from build123d import *

# Parameters (mm, degrees)
BOSS_EXTRUDE1_DEPTH = 17.5
SKETCH2_R           = 1.175
CUT_EXTRUDE1_DEPTH  = 4.41
SKETCH3_R           = 2.75
CUT_EXTRUDE2_DEPTH  = 1


with BuildPart() as part:
    # Sketch1 → Boss-Extrude1 (new body, symmetric)
    with BuildSketch(Plane.XY):
        with BuildLine():
            Line((-3.14, 0.055), (-3.14, -0.055))
            ThreePointArc((-3.14, -0.055), (-3.476827202, -0.868172798), (-4.29, -1.205))
            Line((-4.29, -1.205), (-4.29, -1.705))
            Line((-4.29, -1.705), (4.29, -1.705))
            Line((4.29, -1.705), (4.29, -1.205))
            ThreePointArc((4.29, -1.205), (3.476827202, -0.868172798), (3.14, -0.055))
            Line((3.14, -0.055), (3.14, 0.055))
            ThreePointArc((3.14, 0.055), (3.476827202, 0.868172798), (4.29, 1.205))
            Line((4.29, 1.205), (4.29, 1.705))
            Line((4.29, 1.705), (-4.29, 1.705))
            Line((-4.29, 1.705), (-4.29, 1.205))
            ThreePointArc((-4.29, 1.205), (-3.476827202, 0.868172798), (-3.14, 0.055))
        make_face()
    extrude(amount=BOSS_EXTRUDE1_DEPTH, both=True)

    # Sketch2 → Cut-Extrude1 (cut, through all)
    with BuildSketch(Plane(origin=(0, 1.705, 0), x_dir=(1, 0, 0), z_dir=(0, 1, 0))):
        with Locations((0, 12.5)):
            Circle(SKETCH2_R)
    cut_extrude1 = extrude(amount=-CUT_EXTRUDE1_DEPTH, mode=Mode.SUBTRACT)

    # Sketch3 → Cut-Extrude2 (cut)
    with BuildSketch(Plane(origin=(0, 1.705, 0), x_dir=(1, 0, 0), z_dir=(0, 1, 0))):
        with Locations((0, 12.5)):
            Circle(SKETCH3_R)
    cut_extrude2 = extrude(amount=-CUT_EXTRUDE2_DEPTH, mode=Mode.SUBTRACT)

    # Mirror1: Cut-Extrude1, Cut-Extrude2 across plane
    add(cut_extrude1.mirror(Plane.XY), mode=Mode.SUBTRACT)
    add(cut_extrude2.mirror(Plane.XY), mode=Mode.SUBTRACT)


solid = part.part
Verification items for the finished model (mm, model axes). A direction names the side the tool comes from. Round coordinates to 2 decimals unless told otherwise and drop trailing zeros. Loops run counter-clockwise (first coordinate to the right, second up) from the corner with the lowest first, then second, coordinate; pieces in that order, holes last. Notation, with made-up numbers: (64.5, 28) - (74.5, 28) arc R24 ccw to (74.5, 47) - close; hole circle Ø10 at (49.5, 79). An arc over 180 degrees is marked (long way). Use a Markdown table: item, result. Add a question column.
1. Release check for a two-part mould opening along X. For faces 6 (the face through (0, -1.705, 0)), 7 (the face through (-0.25, -0.48, 11.35)), 8 (the face through (-3.47, -0.86, 0.25)) record: released by +X, released by -X, zero draft, split by the parting line, or undercut.
2. Section check A-A, the plane x = 0. Record the boundary of the cut face in (y, z) (3 decimals).
3. Thickness scan on probe 1 along Z at (x, y) = (0, -0.45) (3 decimals); probe 2 along Z at (x, y) = (0, 1.15); probe 3 along X at (y, z) = (-0.15, 2). Record the ranges inside material, lowest first. Write a range as [from, to].
4. Section check B-B, the plane z = 12.5. Record the boundary of the cut face in (x, y) (3 decimals).
5. Section check D-D, the plane z = 7.5. Record the boundary of the cut face in (x, y) (3 decimals).
6. Section check C-C, the plane y = -0.5. Record the boundary of the cut face in (x, z) (3 decimals).
7. Access from +Z, -Z, +X, -X, +Y, -Y to the whole of each face (thin tool, end or side, straight path). Record for faces 1 (the face through (0, 0.705, -11)), 2 (the face through (0, 1.705, 0)), 3 (the face through (-3.49, 0.88, 0.25)), 4 (the face through (3.47, 0.86, 0.25)), 5 (the face through (-0.25, -0.48, -11.35)).
8. Gauge pin test, flat ends, axial feed: pin 1 (5 mm diameter, centred on x = 0, z = -12.5, fed in from +Y) (3 decimals); pin 2 (1 mm diameter, centred on y = 0, z = 12.5, fed in from -X); pin 3 (1.4 mm diameter, centred on x = 0, z = 12.5, fed in from +Y). Record the tip position at first contact, or that the pin passes through.
Checks:
| question | item | result |
|---|---|---|
| 1 | face 6 | zero draft |
| 1 | face 7 | undercut |
| 1 | face 8 | released by -X |
| 2 | outline | (-1.705, -17.5) - (1.705, -17.5) - (1.705, -15.25) - (0.705, -15.25) - (0.705, -13.675) - (-1.705, -13.675) - close; (-1.705, -11.325) - (0.705, -11.325) - (0.705, -9.75) - (1.705, -9.75) - (1.705, 9.75) - (0.705, 9.75) - (0.705, 11.325) - (-1.705, 11.325) - close; (-1.705, 13.675) - (0.705, 13.675) - (0.705, 15.25) - (1.705, 15.25) - (1.705, 17.5) - (-1.705, 17.5) - close |
| 3 | probe 1 | z = [-17.5, -13.675], [-11.325, 11.325], [13.675, 17.5] |
| 3 | probe 2 | z = [-17.5, -15.25], [-9.75, 9.75], [15.25, 17.5] |
| 3 | probe 3 | x = [-3.14, 3.14] |
| 4 | outline | (-4.29, -1.705) - (-1.175, -1.705) - (-1.175, 0.705) - (-2.75, 0.705) - (-2.75, 1.705) - (-4.29, 1.705) - (-4.29, 1.205) arc R1.15 cw to (-3.14, 0.055) - (-3.14, -0.055) arc R1.15 cw to (-4.29, -1.205) - close; (1.175, -1.705) - (4.29, -1.705) - (4.29, -1.205) arc R1.15 cw to (3.14, -0.055) - (3.14, 0.055) arc R1.15 cw to (4.29, 1.205) - (4.29, 1.705) - (2.75, 1.705) - (2.75, 0.705) - (1.175, 0.705) - close |
| 5 | outline | (-4.29, -1.705) - (4.29, -1.705) - (4.29, -1.205) arc R1.15 cw to (3.14, -0.055) - (3.14, 0.055) arc R1.15 cw to (4.29, 1.205) - (4.29, 1.705) - (-4.29, 1.705) - (-4.29, 1.205) arc R1.15 cw to (-3.14, 0.055) - (-3.14, -0.055) arc R1.15 cw to (-4.29, -1.205) - close |
| 6 | outline | (-3.23, -17.5) - (3.23, -17.5) - (3.23, 17.5) - (-3.23, 17.5) - close; hole circle Ø2.35 at (0, -12.5); hole circle Ø2.35 at (0, 12.5) |
| 7 | face 1 | +Y |
| 7 | face 2 | +Z, -Z, +X, -X, +Y |
| 7 | face 3 | +Z, -Z, -X |
| 7 | face 4 | +Z, -Z, +X |
| 7 | face 5 | +Y, -Y |
| 8 | pin 1 | stops at y = 0.705 |
| 8 | pin 2 | stops at x = -3.23 |
| 8 | pin 3 | passes through |
